from build123d import *

# Parameters (mm, degrees)
SKETCH1_R           = 2.15
SKETCH1_R_2         = 19.1
BOSS_EXTRUDE1_DEPTH = 5
SKETCH2_W           = 57.2
SKETCH2_H           = 57.2
CUT_EXTRUDE1_DEPTH  = 1.5


with BuildPart() as part:
    # Sketch1 → Boss-Extrude1 (new body)
    with BuildSketch(Plane(origin=(0, 0, 0), x_dir=(1, 0, 0), z_dir=(0, 1, 0))):
        Polygon((-25, -55), (25, -55), (55, -25), (55, 25), (25, 55), (-25, 55), (-55, 25), (-55, -25), align=None)
        with Locations(Location((23.57, 23.57, 0), (0, 0, 270))):
            Circle(SKETCH1_R, mode=Mode.SUBTRACT)
        with Locations(Location((-23.57, 23.57, 0), (0, 0, 270))):
            Circle(SKETCH1_R, mode=Mode.SUBTRACT)
        with Locations(Location((-23.57, -23.57, 0), (0, 0, 270))):
            Circle(SKETCH1_R, mode=Mode.SUBTRACT)
        with Locations(Location((23.57, -23.57, 0), (0, 0, 270))):
            Circle(SKETCH1_R, mode=Mode.SUBTRACT)
        with Locations(Location((0, 0, 0), (0, 0, 270))):
            Circle(SKETCH1_R_2, mode=Mode.SUBTRACT)
        with Locations(Location((-8, 50, 0), (0, 0, 270))):
            Circle(SKETCH1_R, mode=Mode.SUBTRACT)
        with Locations(Location((8, 50, 0), (0, 0, 90))):
            Circle(SKETCH1_R, mode=Mode.SUBTRACT)
        with Locations(Location((50, 8, 0), (0, 0, 270))):
            Circle(SKETCH1_R, mode=Mode.SUBTRACT)
        with Locations(Location((50, -8, 0), (0, 0, 90))):
            Circle(SKETCH1_R, mode=Mode.SUBTRACT)
        with Locations(Location((8, -50, 0), (0, 0, 270))):
            Circle(SKETCH1_R, mode=Mode.SUBTRACT)
        with Locations(Location((-8, -50, 0), (0, 0, 90))):
            Circle(SKETCH1_R, mode=Mode.SUBTRACT)
        with Locations(Location((-50, -8, 0), (0, 0, 270))):
            Circle(SKETCH1_R, mode=Mode.SUBTRACT)
        with Locations(Location((-50, 8, 0), (0, 0, 90))):
            Circle(SKETCH1_R, mode=Mode.SUBTRACT)
    extrude(amount=BOSS_EXTRUDE1_DEPTH)

    # Sketch2 → Cut-Extrude1 (cut)
    with BuildSketch(Plane(origin=(0, 5, 0), x_dir=(1, 0, 0), z_dir=(0, 1, 0))):
        Rectangle(SKETCH2_W, SKETCH2_H)
    extrude(amount=-CUT_EXTRUDE1_DEPTH, mode=Mode.SUBTRACT)


solid = part.part
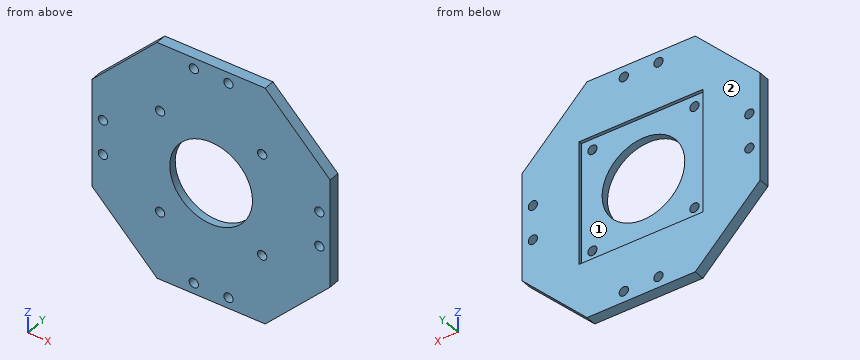
The listing builds one solid part. Answer for the finished solid, in the listing's coordinates (mm). Face numbers are marked on the shaded views. Give positions to 0.01 mm unless a question says otherwise; leave off trailing zeros. Write each loop counter-clockwise with the first axis right and the second up, starting at its lowest first coordinate (ties: lowest second). Pieces come first, ordered by that corner, then holes. Notation, with made-up numbers: (5.5, 73.5) - (22.5, 73.5) arc R16 cw to (22.5, 81.5) - close; hole circle Ø10 at (30, 81.5). An arc over 180 degrees is marked (long way). Use a Markdown table: item, result.
1. Each of these flat-tipped pins is pushed along its axis until it touches: P1, Ø7, axis at x = 23.57, z = 23.57, coming from the +Y side; P2, Ø1, axis at y = 3, z = -26.5, coming from the +X side; P3, Ø1, axis at y = 0.5, z = 43.5, coming from the +X side. Where does it stop, or does it pass through?
Values follow:
| item | result |
|---|---|
| P1 | stops at y = 3.5 |
| P2 | stops at x = 54 |
| P3 | stops at x = 37 |
2. Section A-A on x = -23.57 is taken. Write down the section's boundary in (y, z), plus the area to 3 significant figures.
Values follow:
| item | result |
|---|---|
| outline | (0, -55) - (5, -55) - (5, -28.6) - (3.5, -28.6) - (3.5, -25.72) - (0, -25.72) - close; (0, -21.42) - (3.5, -21.42) - (3.5, 21.42) - (0, 21.42) - close; (0, 25.72) - (3.5, 25.72) - (3.5, 28.6) - (5, 28.6) - (5, 55) - (0, 55) - close |
| area | 434 mm² |
3. Find the intervals of material crossed by probe 1 along X at (y, z) = (2.4, 23.57); probe 2 along X at (y, z) = (3.55, 8), in increasing order. Write a range as from..to.
Values follow:
| item | result |
|---|---|
| probe 1 | x = -55..-25.72, -21.42..21.42, 25.72..55 |
| probe 2 | x = -55..-52.15, -47.85..-28.6, 28.6..47.85, 52.15..55 |
4. Section B-B on x = 0 is taken. Write down the section's boundary in (y, z).
Values follow:
| item | result |
|---|---|
| outline | (0, -55) - (5, -55) - (5, -28.6) - (3.5, -28.6) - (3.5, -19.1) - (0, -19.1) - close; (0, 19.1) - (3.5, 19.1) - (3.5, 28.6) - (5, 28.6) - (5, 55) - (0, 55) - close |
5. Section C-C on y = 1.55 is taken. Count the separate pieces of the cut face and the enclosed holes in it, plus the area to 3 significant figures.
Values follow:
| item | result |
|---|---|
| separate pieces | 1 |
| enclosed holes | 13 |
| area | 8,980 mm² |
6. Section D-D on z = -8 is taken. Write down the section's boundary in (x, y), plus the area to 3 significant figures.
Values follow:
| item | result |
|---|---|
| outline | (-55, 0) - (-52.15, 0) - (-52.15, 5) - (-55, 5) - close; (-47.85, 0) - (-17.34, 0) - (-17.34, 3.5) - (-28.6, 3.5) - (-28.6, 5) - (-47.85, 5) - close; (17.34, 0) - (47.85, 0) - (47.85, 5) - (28.6, 5) - (28.6, 3.5) - (17.34, 3.5) - close; (52.15, 0) - (55, 0) - (55, 5) - (52.15, 5) - close |
| area | 300 mm² |
7. For a pull along X with two mould halves and no side action, classify the marked faces 1 and 2 as released by +X, released by -X, zero draft, split by the parting line, or undercut.
Values follow:
| item | result |
|---|---|
| face 1 | undercut |
| face 2 | zero draft |
